from build123d import *

# Parameters (mm, degrees)
BOSS_EXTRUDE1_DEPTH = 8
BOSS_EXTRUDE4_START = 30
BOSS_EXTRUDE4_DEPTH = 8
SKETCH7_R           = 17.223036208
BOSS_EXTRUDE5_DEPTH = 38
SKETCH8_R           = 17
BOSS_EXTRUDE6_DEPTH = 35
BOSS_EXTRUDE7_START = 35
SKETCH9_R           = 17
BOSS_EXTRUDE7_DEPTH = 35


with BuildPart() as part:
    # Sketch1 → Boss-Extrude1 (new body)
    with BuildSketch(Plane.XY):
        with BuildLine():
            Line((-12.5, 21.650635095), (39.461524227, 51.650635095))
            Line((39.461524227, 51.650635095), (39.461524227, 86.650635095))
            ThreePointArc((39.461524227, 86.650635095), (126.112159322, 0), (39.461524227, -86.650635095))
            Line((39.461524227, -86.650635095), (39.461524227, -51.650635095))
            Line((39.461524227, -51.650635095), (-12.5, -21.650635095))
            ThreePointArc((-12.5, -21.650635095), (-25, 0), (-12.5, 21.650635095))
        make_face()
    extrude(amount=BOSS_EXTRUDE1_DEPTH)



with BuildPart() as body_2:
    # Sketch5 → Boss-Extrude4 (new body)
    with BuildSketch(Plane(origin=(0, 0, 0), x_dir=(-1, 0, 0), z_dir=(0, 0, -1)).offset(BOSS_EXTRUDE4_START)):
        with BuildLine():
            Line((-39.461524227, 86.650635095), (-39.461524227, 51.650635095))
            Line((-39.461524227, 51.650635095), (12.5, 21.650635095))
            ThreePointArc((12.5, 21.650635095), (25, 0), (12.5, -21.650635095))
            Line((12.5, -21.650635095), (-39.461524227, -51.650635095))
            Line((-39.461524227, -51.650635095), (-39.461524227, -86.650635095))
            ThreePointArc((-39.461524227, -86.650635095), (-126.112159322, 0), (-39.461524227, 86.650635095))
        make_face()
    extrude(amount=BOSS_EXTRUDE4_DEPTH)


with BuildPart() as part_1:
    add(part.part)

    add(body_2.part)  # Boss-Extrude5 merges body 2
    # Sketch7 → Boss-Extrude5 (add)
    with BuildSketch(Plane.XY.offset(8)):
        Circle(SKETCH7_R)
    extrude(amount=-BOSS_EXTRUDE5_DEPTH)

    # Sketch8 → Boss-Extrude6 (add)
    with BuildSketch(Plane.XY.offset(8)):
        with Locations((39.461524227, 0)):
            Circle(SKETCH8_R)
    extrude(amount=BOSS_EXTRUDE6_DEPTH)

    # Sketch9 → Boss-Extrude7 (add)
    with BuildSketch(Plane(origin=(0, 0, -38), x_dir=(-1, 0, 0), z_dir=(0, 0, -1)).offset(BOSS_EXTRUDE7_START)):
        with Locations(Location((-39.461524227, 0, 0), (0, 0, 180))):
            Circle(SKETCH9_R)
    extrude(amount=-BOSS_EXTRUDE7_DEPTH)


solid = part_1.part
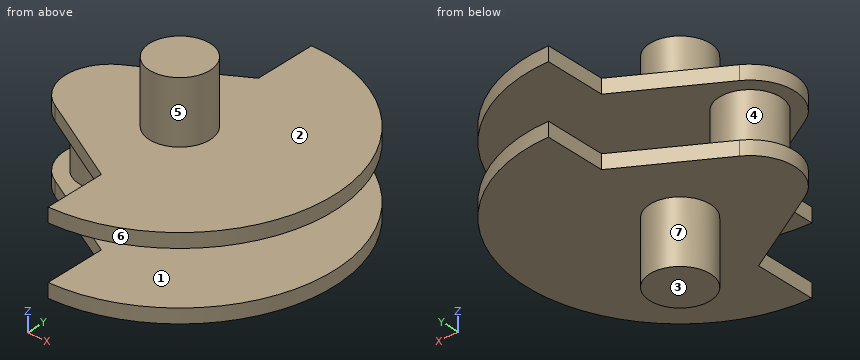
The listing builds one solid part. Answer for the finished solid, in the listing's coordinates (mm). Face numbers are marked on the shaded views. A direction names the side the tool comes from. Give positions to 0.01 mm unless a question says otherwise; leave off trailing zeros. Write each loop counter-clockwise with the first axis right and the second up, starting at its lowest first coordinate (ties: lowest second). Pieces come first, ordered by that corner, then holes. Notation, with made-up numbers: (21, 55) - (79, 55) arc R18 ccw to (79, 74) - close; hole circle Ø4 at (16.5, -11.5). An arc over 180 degrees is marked (long way). One line per question, with ' | ' between items. Start each with the question number.
1. Determine the mould class of the marked faces 1, 2 and 3 for opening direction Z: +Z half, -Z half, draft (parallel to the pull), parting line (faces both ways), or undercut.
2. Section D-D, the plane z = -12 is taken. Determine the outline of the cut face in (x, y), then the cut area to 3 significant figures.
3. For the marked faces 4, 5, 6 and 7, determine the directions among +Z, -Z, +X, -X, +Y, -Y from which every point of the face is accessible in a straight line to the end or side of a thin tool.
4. Section C-C, the plane y = 68 is taken. Determine the outline of the cut face in (x, z).
5. Section A-A, the plane x = 76 is taken. Determine the outline of the cut face in (y, z), then the cut area to 3 significant figures.
6. Straight lines are drawn through the part: line 1 (Z direction, x = 80, y = -68); line 2 (Z direction, x = 53, y = 0.5); line 3 (Y direction, x = 39.5, z = -58). For each, find the intervals that lie inside material, in ascending order.
7. Given P1, Ø2.5, axis at y = 69.5, z = -33, coming from the -X side; P2, Ø10, axis at x = 87, y = 9, coming from the -Z side; P3, Ø12, axis at y = 13, z = 21, coming from the -X side, each flat-ended and moving along its own axis, determine where each tip first touches the part or whether it passes through.
8. Section B-B, the plane y = 0 is taken. Determine the outline of the cut face in (x, z).
Result:
1) face 1: undercut | face 2: +Z half | face 3: -Z half
2) outline: circle Ø34.45 at (0, 0) | area: 932 mm2
3) face 4: none | face 5: +Z | face 6: +Z, -Z, +X | face 7: -Z
4) outline: (39.46, -38) - (93.17, -38) - (93.17, -30) - (39.46, -30) - close; (39.46, 0) - (93.17, 0) - (93.17, 8) - (39.46, 8) - close
5) outline: (-78.57, -38) - (78.57, -38) - (78.57, -30) - (-78.57, -30) - close; (-78.57, 0) - (78.57, 0) - (78.57, 8) - (-78.57, 8) - close | area: 2,510 mm2
6) line 1: z = -38 to -30, 0 to 8 | line 2: z = -73 to -30, 0 to 43 | line 3: y = -17 to 17
7) P1: stops at x = 39.46 | P2: stops at z = -38 | P3: stops at x = 23.97
8) outline: (-25, -38) - (22.46, -38) - (22.46, -73) - (56.46, -73) - (56.46, -38) - (126.11, -38) - (126.11, -30) - (17.22, -30) - (17.22, 0) - (126.11, 0) - (126.11, 8) - (56.46, 8) - (56.46, 43) - (22.46, 43) - (22.46, 8) - (-25, 8) - (-25, 0) - (-17.22, 0) - (-17.22, -30) - (-25, -30) - close
